The listing builds one solid part. Answer for the finished solid, in the listing's coordinates (mm). A direction names the side the tool comes from. Coordinates: 2 decimals unless noted, no trailing zeros. Write each loop counter-clockwise with the first axis right and the second up, starting at its lowest first coordinate (ties: lowest second). Pieces come first, ordered by that corner, then holes. Notation, with made-up numbers: M 32.25,-1 L 39.25,-1 A31 ccw 39.25,23 Z; hole C 51.25,34 d8. An arc over 180 degrees is marked long. Answer as a JSON object with one key per item and string values. Group by question number.
from build123d import *

# Parameters (mm, degrees)
SKETCH1_W           = 80
SKETCH1_H           = 50
BOSS_EXTRUDE1_DEPTH = 2.5
SKETCH2_W           = 80
SKETCH2_H           = 50
SKETCH2_W_2         = 75
SKETCH2_H_2         = 45
BOSS_EXTRUDE2_DEPTH = 37.5
CUT_EXTRUDE2_DEPTH  = 2.5
SKETCH11_W          = 80
SKETCH11_H          = 50
CUT_EXTRUDE10_DEPTH = 0.1
BOSS_EXTRUDE4_DEPTH = 5
SKETCH8_W           = 10
SKETCH8_H           = 7
CUT_EXTRUDE14_DEPTH = 10
SKETCH15_W          = 75
SKETCH15_H          = 37.5
CUT_EXTRUDE15_DEPTH = 10
SKETCH14_W          = 22.5
SKETCH14_H          = 22
CUT_EXTRUDE16_DEPTH = 2.5


with BuildPart() as part:
    # Sketch1 → Boss-Extrude1 (new body)
    with BuildSketch(Plane(origin=(0, 0, 0), x_dir=(1, 0, 0), z_dir=(0, 1, 0))):
        with Locations((-26.709650323, 17.072563556)):
            Rectangle(SKETCH1_W, SKETCH1_H)
    extrude(amount=BOSS_EXTRUDE1_DEPTH)

    # Sketch2 → Boss-Extrude2 (add)
    with BuildSketch(Plane(origin=(0, 2.5, 0), x_dir=(1, 0, 0), z_dir=(0, 1, 0))):
        with Locations((-26.709650323, 17.072563556)):
            Rectangle(SKETCH2_W, SKETCH2_H)
        with Locations((-26.709650323, 17.072563556)):
            Rectangle(SKETCH2_W_2, SKETCH2_H_2, mode=Mode.SUBTRACT)
    extrude(amount=BOSS_EXTRUDE2_DEPTH)

    # Sketch5 → Cut-Extrude2 (cut)
    with BuildSketch(Plane.XY.offset(7.927436444)):
        with BuildLine():
            Line((-20.404890216, 2.5), (-33.014410429, 2.5))
            ThreePointArc((-33.014410429, 2.5), (-26.709650323, 29), (-20.404890216, 2.5))
        make_face()
    extrude(amount=-CUT_EXTRUDE2_DEPTH, mode=Mode.SUBTRACT)

    # Sketch11 → Cut-Extrude10 (cut)
    with BuildSketch(Plane(origin=(0, 0, 0), x_dir=(-1, 0, 0), z_dir=(0, -1, 0))):
        with Locations((26.709650323, 17.072563556)):
            Rectangle(SKETCH11_W, SKETCH11_H)
    extrude(amount=-CUT_EXTRUDE10_DEPTH, mode=Mode.SUBTRACT)

    # Sketch6 → Boss-Extrude4 (add)
    with BuildSketch(Plane(origin=(0, 2.5, 0), x_dir=(1, 0, 0), z_dir=(0, 1, 0))):
        Polygon((-40.709650323, 39.572563556), (-12.709650323, 39.572563556), (-12.709650323, 14.572563556), (-18.209650323, 14.572563556), (-18.209650323, 34.072563556), (-35.209650323, 34.072563556), (-35.209650323, 14.572563556), (-40.709650323, 14.572563556), align=None)
    extrude(amount=BOSS_EXTRUDE4_DEPTH)

    # Sketch8 → Cut-Extrude14 (cut)
    with BuildSketch(Plane(origin=(0, 2.5, 0), x_dir=(1, 0, 0), z_dir=(0, 1, 0))):
        with Locations((-26.709650323, 18.072563556)):
            Rectangle(SKETCH8_W, SKETCH8_H)
    extrude(amount=-CUT_EXTRUDE14_DEPTH, mode=Mode.SUBTRACT)

    # Sketch15 → Cut-Extrude15 (cut)
    with BuildSketch(Plane(origin=(0, 0, 5.427436444), x_dir=(-1, 0, 0), z_dir=(0, 0, -1))):
        with Locations((26.709650323, 21.25)):
            Rectangle(SKETCH15_W, SKETCH15_H)
    extrude(amount=-CUT_EXTRUDE15_DEPTH, mode=Mode.SUBTRACT)

    # Sketch14 → Cut-Extrude16 (cut)
    with BuildSketch(Plane(origin=(0, 7.5, 0), x_dir=(1, 0, 0), z_dir=(0, 1, 0))):
        with Locations((-26.709650323, 25.572563556)):
            Rectangle(SKETCH14_W, SKETCH14_H)
    extrude(amount=-CUT_EXTRUDE16_DEPTH, mode=Mode.SUBTRACT)


solid = part.part
Item 1: A cutting plane is placed at D-D, the plane z = -3.5. Write down the section's boundary in (x, y).
Item 2: A cutting plane is placed at A-A, the plane z = -23.5. Write down the section's boundary in (x, y).
Item 3: A tool of negligible diameter and unlimited length cuts with its end or side. For faces 1 (the face through (-66.71, 20, -17)), 2 (the face through (-21.71, 1, -18)), 3 (the face through (-35.21, 4, -24)), from which of +Z, -Z, +X, -X, +Y, -Y can it reach the whole face along a straight path? Write none if from no direction.
Item 4: Flat-ended cylindrical pins translate along their axes: pin 1 Ø1.2 at (x, y) = (-26, 3) entering from +Z; pin 2 Ø1.5 at (x, y) = (-42, 31) entering from +Z; pin 3 Ø6.5 at (x, z) = (-24.5, -27) entering from +Y; pin 4 Ø4 at (x, y) = (-14, 5) entering from +Z. Find the tip coordinate at first contact, or state that the pin passes through.
Item 5: Consider L1, parallel to X at y = 3, z = -23; L2, parallel to X at y = 5, z = -7; L3, parallel to Z at x = -24, y = 2. Determine where each line is inside the solid, lowest interval first. Write a range as from..to.
Item 6: A cutting plane is placed at C-C, the plane x = 1. Write down the section's boundary in (y, z), and give its area (3 significant figures).
Item 7: For a pull along Z with two mould halves and no side action, classify faces 4 (the face through (-27, 1, -21.573)), 5 (the face through (-27, 20, -42.073)), 6 (the face through (-28, 5, -35)), 7 (the face through (-39, 4, -14.573)) as +Z half, -Z half, draft (parallel to the pull), parting line (faces both ways), or undercut.
Item 8: A cutting plane is placed at B-B, the plane y = 25. Write down the section's boundary in (x, z), and give its area (4 significant figures).
Answer:
{
 "1": {"outline": "M -66.71,0.1 L 13.29,0.1 L 13.29,40 L 10.79,40 L 10.79,2.5 L -64.21,2.5 L -64.21,40 L -66.71,40 Z"},
 "2": {"outline": "M -66.71,0.1 L 13.29,0.1 L 13.29,40 L 10.79,40 L 10.79,2.5 L -12.71,2.5 L -12.71,7.5 L -15.46,7.5 L -15.46,5 L -18.21,5 L -18.21,2.5 L -35.21,2.5 L -35.21,5 L -37.96,5 L -37.96,7.5 L -40.71,7.5 L -40.71,2.5 L -64.21,2.5 L -64.21,40 L -66.71,40 Z"},
 "3": {"face 1": "+Z, -Z, -X, +Y, -Y", "face 2": "+Y, -Y", "face 3": "+Z, +Y"},
 "4": {"pin 1": "z = 7.93", "pin 2": "z = -39.57", "pin 3": "y = 2.5", "pin 4": "z = -14.57"},
 "5": {"L1": "-66.71..-64.21, -40.71..-35.21, -18.21..-12.71, 10.79..13.29", "L2": "-66.71..-64.21, 10.79..13.29", "L3": "-42.07..-21.57, -14.57..7.93"},
 "6": {"outline": "M 0.1,-42.07 L 40,-42.07 L 40,-39.57 L 2.5,-39.57 L 2.5,7.93 L 0.1,7.93 Z", "area": "214 mm2"},
 "7": {"face 4": "undercut", "face 5": "-Z half", "face 6": "draft", "face 7": "+Z half"},
 "8": {"outline": "M -66.71,-42.07 L 13.29,-42.07 L 13.29,7.93 L 10.79,7.93 L 10.79,-39.57 L -64.21,-39.57 L -64.21,7.93 L -66.71,7.93 Z", "area": "437.5 mm2"}
}
